Autodesk Inventor part; units mm, degrees
ref_plane "YZ Plane" through (0, 0, 0) normal (1, 0, 0) x (0, 1, 0)
ref_plane "XZ Plane" through (0, 0, 0) normal (0, 1, 0) x (-1, 0, 0)
ref_plane "XY Plane" through (0, 0, 0) normal (0, 0, 1) x (1, 0, 0)
sketch "Sketch1" plane through (0, 0, 0) normal (1, 0, 0) x (0, 1, 0)
  line L0 (0, 11.5) -> (56, 11.5)
  line L1 (56, 11.5) -> (56, -11.5)
  line L2 (56, -11.5) -> (0, -11.5)
  line L3 (0, -11.5) -> (0, 11.5)
  point P0 (0, 0)
  dimension "d0" = 0
  dimension "d1" = 23
  dimension "d2" = 56
  dimension "d3" = 11.5
extrude "Extrusion1" add sketch "Sketch1" along normal mid plane 8
sketch "Sketch2" plane through (4, 0, 0) normal (1, 0, 0) x (0, 0, -1)
  line L0 (11.5, 56) -> (-11.5, 56)
  line L1 (-6.5, 56) -> (6.5, 56)
  line L2 (6.5, 56) -> (6.5, 43)
  line L3 (6.5, 43) -> (-6.5, 43)
  line L4 (-6.5, 43) -> (-6.5, 56)
  point P0 (0, 0)
  dimension "d6" = 13
  dimension "d7" = 13
  dimension "d8" = 6.5
extrude "Extrusion2" cut sketch "Sketch2" against normal through all
sketch "Sketch4" plane through (-4, 0, 11.5) normal (0, 0, 1) x (1, 0, 0)
  circle A0 centre (4, 51) radius 1.5
  line L0 (0, 56) -> (8, 56)
  line L1 (0, 0) -> (8, 0)
  point P0 (4, 0)
  point P1 (4, 0)
  dimension "d12" = 3
  dimension "d13" = 5
hole "Hole1" at (0, 51, 11.5) direction (0, 0, -1) diameter 3 end through all
sketch "Sketch5" plane through (-4, 0, -11.5) normal (0, -1, 0) x (1, 0, 0)
  circle A0 centre (4, 16.5) radius 1.5
  circle A1 centre (4, 6.5) radius 1.5
  point P0 (4, 11.5)
  dimension "d21" = 3
  dimension "d23" = 10
  dimension "d24" = 5
hole "Hole2" at (0, 0, 5) at (0, 0, -5) direction (0, 1, 0) diameter 2.459 depth 13 tip angle 118
sketch "Sketch6" plane through (-4, 0, 11.5) normal (0, 0, 1) x (1, 0, 0)
  circle A0 centre (4, 33) radius 1.5
  circle A1 centre (4, 23) radius 1.5
  line L0 (0, 0) -> (8, 0)
  point P0 (4, 0)
  point P1 (4, 0)
  dimension "d32" = 3
  dimension "d33" = 10
  dimension "d34" = 23
hole "Hole3" at (0, 33, 11.5) at (0, 23, 11.5) direction (0, 0, -1) diameter 2.459 end through all
properties part number "Gripper_Outer_Support" material "Aluminum 6061"
Geometry check sheet. Reference: the model listing, model coordinates, mm. A direction names the side the tool comes from. Coordinates: 2 decimals unless noted, no trailing zeros. Order: outer loops, then holes, each group sorted by start corner. A loop starts at its lowest first (then second) coordinate and runs counter-clockwise, first axis right, second up. Notation, with made-up numbers: (42, -31) - (75, -31) arc R17 cw to (75, -12) - close; hole circle Ø1 at (-16, -7). An arc over 180 degrees is marked (long way). Use one line per item in the form item = value.
1. Section check C-C (z = 2.5). Record the boundary of the cut face in (x, y).
Here are the results:
outline = (-4, 0) - (4, 0) - (4, 43) - (-4, 43) - close; hole circle Ø2.46 at (0, 23); hole circle Ø2.46 at (0, 33)
2. Gauge pin test, flat ends, axial feed: pin 1 (2.5 mm diameter, centred on x = 1, y = 51, fed in from +Z); pin 2 (1.5 mm diameter, centred on x = -2, z = -3.5, fed in from +Y); pin 3 (2 mm diameter, centred on x = 0, z = -5, fed in from -Y). Record the tip position at first contact, or that the pin passes through.
Here are the results:
pin_1 = 11.5
pin_2 = 43
pin_3 = 13.14
3. Access from +Z, -Z, +X, -X, +Y, -Y to the whole of each face (thin tool, end or side, straight path). Record for faces 1 (the face through (-0.05, 6.59, 6.23)), 2 (the face through (0.9, 49.6, -6.5)), 3 (the face through (-0.05, 34.23, -0.16)).
Here are the results:
face_1 = -Y
face_2 = +X, -X, +Y
face_3 = +Z, -Z
4. Draft check along Z on faces 4 (the face through (-4, 28, 0)), 5 (the face through (0, 28, -11.5)), 6 (the face through (-0.05, 6.59, -3.77)). Enter one of: pulls with the +Z half, pulls with the -Z half, needs draft (parallel to the pull), parting line crosses it, or undercut.
Here are the results:
face_4 = needs draft
face_5 = pulls with the -Z half
face_6 = undercut
5. Section check B-B (z = -7). Record the boundary of the cut face in (x, y).
Here are the results:
outline = (-4, 0) - (4, 0) - (4, 56) - (-4, 56) - close; hole circle Ø3 at (0, 51); hole circle Ø2.46 at (0, 23); hole circle Ø2.46 at (0, 33)
6. Scan lines: line 1 (Y direction, x = 0, z = -3); line 2 (Y direction, x = 0, z = -7.7); line 3 (X direction, y = 5, z = -5). Record each from-to range of solid material in increasing order.
Here are the results:
line_1 = 0 to 21.77, 24.23 to 31.77, 34.23 to 43
line_2 = 0 to 21.77, 24.23 to 31.77, 34.23 to 49.5, 52.5 to 56
line_3 = -4 to -1.23, 1.23 to 4
7. Section check A-A (y = 23). Record the boundary of the cut face in (x, z).
Here are the results:
outline = (-4, -11.5) - (-1.23, -11.5) - (-1.23, 11.5) - (-4, 11.5) - close; (1.23, -11.5) - (4, -11.5) - (4, 11.5) - (1.23, 11.5) - close
8. Section check D-D (y = 51). Record the boundary of the cut face in (x, z), then the cut area to 3 significant figures.
Here are the results:
outline = (-4, -11.5) - (-1.5, -11.5) - (-1.5, -6.5) - (-4, -6.5) - close; (-4, 6.5) - (-1.5, 6.5) - (-1.5, 11.5) - (-4, 11.5) - close; (1.5, -11.5) - (4, -11.5) - (4, -6.5) - (1.5, -6.5) - close; (1.5, 6.5) - (4, 6.5) - (4, 11.5) - (1.5, 11.5) - close
area = 50.0 mm²
